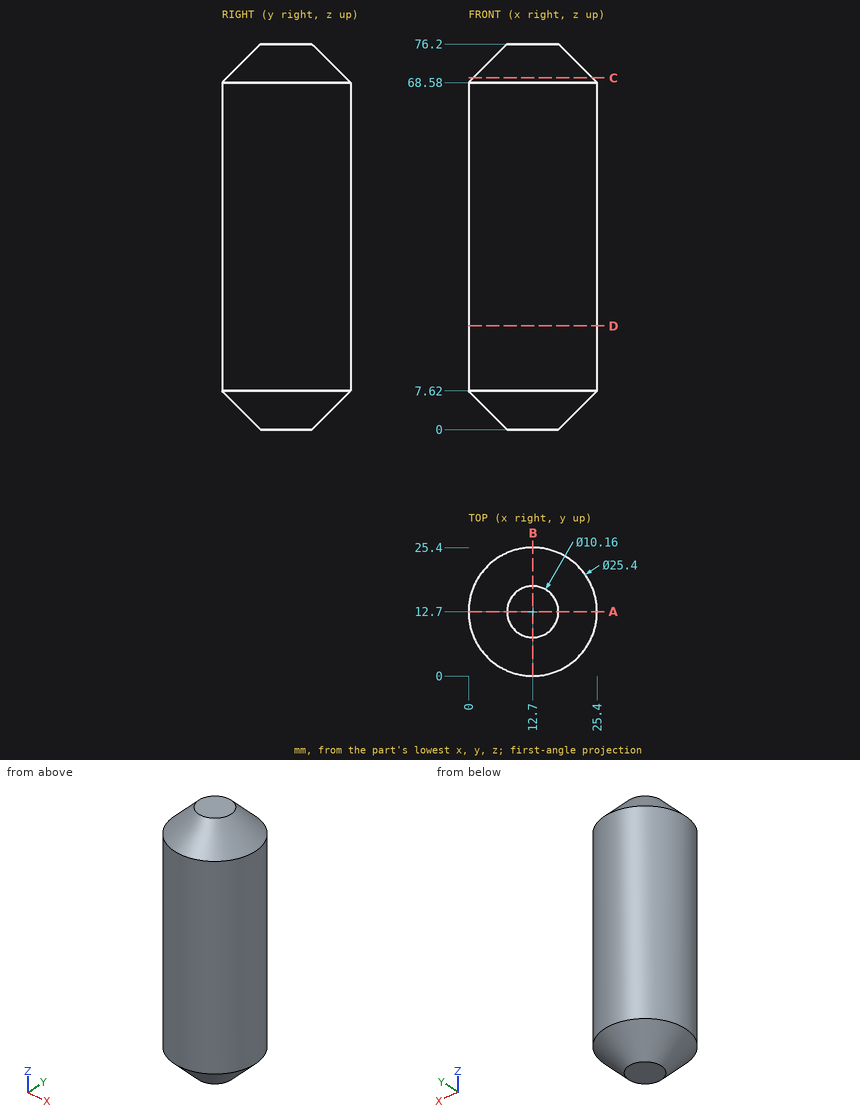
Design review of the part shown in the three views and the two pictorial views. Dimensions are in mm from the part's minimum x, y and z. Round coordinates to 2 decimals unless told otherwise and drop trailing zeros. Loops run counter-clockwise (first coordinate to the right, second up) from the corner with the lowest first, then second, coordinate; pieces in that order, holes last. Notation, with made-up numbers: M -3,36.5 L 35,36.5 A20 ccw 35,56.5 Z; hole C -9,35 d11. An arc over 180 degrees is marked long. Answer as a JSON object with one key per item and string values.
Item 1: For line 1 along X through (y, z) = (10.5, 46); line 2 along Y through (x, z) = (22.5, 64.5); line 3 along Z through (x, y) = (6, 4.25), list the stretches that pass through material, from the lowest coordinate up.
Check sheet entries:
{"line 1": "0.19 to 25.21", "line 2": "4.62 to 20.78", "line 3": "5.7 to 70.5"}
Item 2: We need section C-C, the plane z = 69.5. State the section outline as (x, y) points, and give its area (3 significant figures).
Check sheet entries:
{"outline": "C 12.7,12.7 d23.56", "area": "436 mm2"}
Item 3: We need section D-D, the plane z = 20.5. State the section outline as (x, y) points.
Check sheet entries:
{"outline": "C 12.7,12.7 d25.4"}
Item 4: We need section A-A, the plane y = 12.7. State the section outline as (x, z) points, and give its area (3 significant figures).
Check sheet entries:
{"outline": "M 0,7.62 L 7.62,0 L 17.78,0 L 25.4,7.62 L 25.4,68.58 L 17.78,76.2 L 7.62,76.2 L 0,68.58 Z", "area": "1,820 mm2"}
Item 5: Clearance check with flat-ended pins moving along their axes: P1, Ø2, axis at y = 19.5, z = 24, coming from the +X side; P2, Ø10, axis at x = 18, z = 57, coming from the -Y side; P3, Ø10, axis at x = 6.5, y = 4, coming from the -Z side; P4, Ø8, axis at x = 11.5, z = 48.5, coming from the +Y side. State where each tip first meets the part, or that it passes through.
Check sheet entries:
{"P1": "x = 24", "P2": "y = 0", "P3": "z = 0.6", "P4": "y = 25.4"}
